Input: part model. Units: mm. Frame: model coordinates. Face numbers are marked on the shaded views. Round coordinates to 2 decimals unless told otherwise and drop trailing zeros. Loops run counter-clockwise (first coordinate to the right, second up) from the corner with the lowest first, then second, coordinate; pieces in that order, holes last.
(1) Draft query along Z for the marked faces 1 and 2. Return one class per face: released by +Z, released by -Z, zero draft, split by the parting line, or undercut.
(2) First-contact query: pin 1 Ø8 at (x, z) = (0, 28.5) entering from -Y; pin 2 Ø4.5 at (x, z) = (30, 0) entering from +Y. Flat tips, straight axial feed; report the tip coordinate or a pass-through.
(3) Cut plane C-C, the plane x = 30. Output: boundary loops of the cut face in (y, z) (1 decimal), and give its area (3 significant figures).
(4) Cut plane B-B, the plane x = 0. Output: boundary loops of the cut face in (y, z) (3 decimals).
(5) Cut plane D-D, the plane y = 3.5. Give the number of separate pieces and of enclosed holes in the cut face, and give its area (3 significant figures).
(6) Cut plane A-A, the plane z = -30. Output: boundary loops of the cut face in (x, y) (1 decimal), and give its area (3 significant figures).
(7) Line query: line 1 (Z direction, x = 30, y = 4) (1 decimal); line 2 (Z direction, x = -30, y = 2.5) (1 decimal). Output: solid intervals per line, ascending.
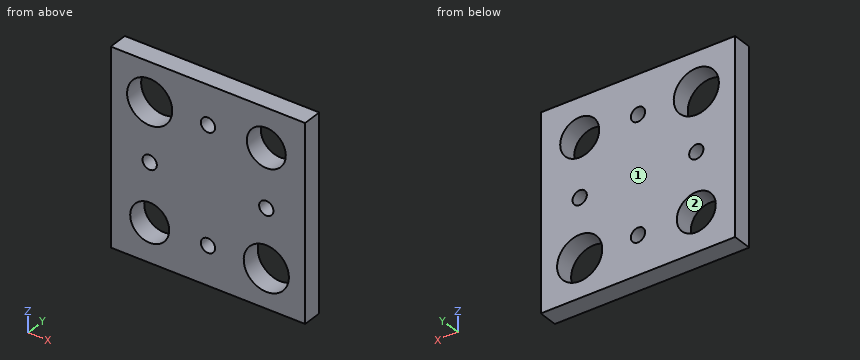
from build123d import *

# Parameters (mm, degrees)
SKETCH1_W               = 100
SKETCH1_H               = 100
BOSS_EXTRUDE1_DEPTH     = 10
CUT_EXTRUDE3_DEPTH      = 72.414284285
CUT_EXTRUDE3_DEPTH_BACK = 72.414284285
SKETCH3_R               = 10.025
SKETCH3_R_2             = 3.675
SKETCH3_R_3             = 11.6125


with BuildPart() as part:
    # Sketch1 → Boss-Extrude1 (new body)
    with BuildSketch(Plane(origin=(0, 0, 0), x_dir=(1, 0, 0), z_dir=(0, 1, 0))):
        Rectangle(SKETCH1_W, SKETCH1_H)
    extrude(amount=BOSS_EXTRUDE1_DEPTH)

    # Sketch3 → Cut-Extrude3 (cut, two sides: drawn at the far end of the back side and taken through both)
    with BuildSketch(Plane(origin=(0, 0, 0), x_dir=(1, 0, 0), z_dir=(0, 1, 0)).offset(-CUT_EXTRUDE3_DEPTH_BACK)):
        with Locations(Location((-30, 30, 0), (0, 0, 270))):
            Circle(SKETCH3_R)
        with Locations(Location((30, -30, 0), (0, 0, 270))):
            Circle(SKETCH3_R)
        with Locations(Location((0, 30, 0), (0, 0, 270))):
            Circle(SKETCH3_R_2)
        with Locations(Location((30, 0, 0), (0, 0, 270))):
            Circle(SKETCH3_R_2)
        with Locations(Location((0, -30, 0), (0, 0, 270))):
            Circle(SKETCH3_R_2)
        with Locations(Location((-30, 0, 0), (0, 0, 270))):
            Circle(SKETCH3_R_2)
        with Locations(Location((30, 30, 0), (0, 0, 270))):
            Circle(SKETCH3_R_3)
        with Locations(Location((-30, -30, 0), (0, 0, 270))):
            Circle(SKETCH3_R_3)
    extrude(amount=CUT_EXTRUDE3_DEPTH + CUT_EXTRUDE3_DEPTH_BACK, mode=Mode.SUBTRACT)


solid = part.part
Reported:
1. face 1: zero draft
1. face 2: undercut
2. pin 1: stops at y = 0
2. pin 2: passes through
3. outline: (0, -50) - (10, -50) - (10, -41.6) - (0, -41.6) - close; (0, -18.4) - (10, -18.4) - (10, -3.7) - (0, -3.7) - close; (0, 3.7) - (10, 3.7) - (10, 20) - (0, 20) - close; (0, 40) - (10, 40) - (10, 50) - (0, 50) - close
3. area: 494 mm2
4. outline: (0, -50) - (10, -50) - (10, -33.675) - (0, -33.675) - close; (0, -26.325) - (10, -26.325) - (10, 26.325) - (0, 26.325) - close; (0, 33.675) - (10, 33.675) - (10, 50) - (0, 50) - close
5. separate pieces: 1
5. enclosed holes: 8
5. area: 8,350 mm2
6. outline: (-50, 0) - (-40, 0) - (-40, 10) - (-50, 10) - close; (-20, 0) - (-3.7, 0) - (-3.7, 10) - (-20, 10) - close; (3.7, 0) - (18.4, 0) - (18.4, 10) - (3.7, 10) - close; (41.6, 0) - (50, 0) - (50, 10) - (41.6, 10) - close
6. area: 494 mm2
7. line 1: z = -50 to -41.6, -18.4 to -3.7, 3.7 to 20, 40 to 50
7. line 2: z = -50 to -40, -20 to -3.7, 3.7 to 18.4, 41.6 to 50
